Autodesk Inventor part; units mm, degrees
ref_plane "YZ Plane" through (0, 0, 0) normal (1, 0, 0) x (0, 1, 0)
ref_plane "XZ Plane" through (0, 0, 0) normal (0, 1, 0) x (-1, 0, 0)
ref_plane "XY Plane" through (0, 0, 0) normal (0, 0, 1) x (1, 0, 0)
sketch "スケッチ1" plane through (0, 0, 0) normal (0, 0, 1) x (1, 0, 0)
  circle A0 centre (0, 0) radius 48.5
  circle A1 centre (0, 0) radius 46
  dimension "d0" = 97
  dimension "d1" = 92
extrude "押し出し1" add sketch "スケッチ1" along normal blind 20.5 contours A0 | A1
sketch "スケッチ2" plane through (0, 0, 20.5) normal (0, 0, 1) x (1, 0, 0)
  circle A0 centre (0, 0) radius 46
  line L0 (0, 0) -> (0, 59.211017)
  line L1 (0, 0) -> (-21.860946, 52.776992)
  line L2 (0, 0) -> (27.822621, 47.858094)
  point P0 (-17.603438, 42.498458)
  point P1 (-42.498458, 17.603438)
  point P2 (-42.498458, -17.603438)
  point P3 (-17.603438, -42.498458)
  point P4 (17.603438, -42.498458)
  point P5 (42.498458, -17.603438)
  point P6 (42.498458, 17.603438)
  point P7 (17.603438, 42.498458)
  dimension "d4" = 92
  dimension "d5" = 22.5
  dimension "d8" = 360
hole "穴1" at (-17.603438, 42.498458, 20.5) at (-42.498458, 17.603438, 20.5) at (-42.498458, -17.603438, 20.5) at (-17.603438, -42.498458, 20.5) at (17.603438, -42.498458, 20.5) at (42.498458, -17.603438, 20.5) at (42.498458, 17.603438, 20.5) at (17.603438, 42.498458, 20.5) direction (0, 0, -1) diameter 2.459 end through all
sketch "スケッチ3" plane through (0, 0, 20.5) normal (0, 0, 1) x (1, 0, 0)
  circle A0 centre (0, 0) radius 43.5
  dimension "d17" = 87
extrude "押し出し2" cut sketch "スケッチ3" against normal blind 20
sketch "スケッチ4" plane through (0, 0, 0) normal (0, 0, -1) x (-1, 0, 0)
  line L0 (0, 0) -> (0, -80.557014)
  circle A0 centre (0, 0) radius 48.5
  line L1 (-29.457728, -38.529109) -> (145.313488, -172.151794)
  line L2 (29.457728, 38.529109) -> (204.228945, -95.093576)
  line L3 (145.313488, -172.151794) -> (204.228945, -95.093576)
  point P0 (29.457728, 38.529109)
  dimension "d21" = 48.5
  dimension "d23" = 97
  dimension "d24" = 220
  dimension "d25" = 220
  dimension "d56" = 52.6
extrude "押し出し3" add sketch "スケッチ4" against normal blind 5 contours A0 L2 L3 L1 L0 | L0 L1 A0
sketch "スケッチ5" plane through (0, 0, 5) normal (0, 0, 1) x (1, 0, 0)
  line L0 (-29.457728, 38.529109) -> (29.457728, -38.529109)
  line L1 (-204.228945, -95.093576) -> (-145.313488, -172.151794)
  line L2 (29.457728, -38.529109) -> (-145.313488, -172.151794)
  line L3 (-145.313488, -172.151794) -> (-204.228945, -95.093576)
  line L4 (-204.228945, -95.093576) -> (-29.457728, 38.529109)
  line L5 (-26.420849, 34.557036) -> (-201.192066, -99.065649)
  line L6 (26.420849, -34.557036) -> (-148.350367, -168.179721)
  line L7 (-200.256872, -92.056696) -> (-141.341415, -169.114915)
  circle A0 centre (0, 0) radius 48.5
  circle A1 centre (0, 0) radius 43.5
  point P0 (-116.843336, -28.282233)
  point P1 (-60.964759, -101.368378)
  point P2 (-57.92788, -105.340451)
  point P3 (-174.771217, -133.622685)
  point P4 (-170.799143, -130.585806)
  point P5 (-174.771217, -133.622685)
  point P6 (-43.459144, 21.530276)
  point P7 (9.382554, -47.583796)
  point P8 (-144.378294, -165.142842)
  point P9 (-197.219992, -96.02877)
  dimension "d29" = 5
  dimension "d30" = 5
  dimension "d32" = 5
  dimension "d33" = 5
extrude "押し出し4" add sketch "スケッチ5" along normal blind 15.5 contours A0 L5 L7 L4 | L7 L5 L1 L4 | L7 L6 L1 L5 | L2 L7 L6 A0 | L7 L2 L1 L6
sketch "スケッチ6" plane through (0, 0, 20.5) normal (0, 0, 1) x (1, 0, 0)
  line L0 (-204.228945, -95.093576) -> (-145.313488, -172.151794)
  arc A0 (29.457728, -38.529109) -> (-29.457728, 38.529109) centre (0, 0) ccw
  line L1 (-29.457728, 38.529109) -> (-204.228945, -95.093576)
  line L2 (-145.313488, -172.151794) -> (29.457728, -38.529109)
  point P0 (-15.753516, -69.948744)
  point P1 (-71.632093, 3.137401)
  point P2 (-59.44632, -103.354415)
  point P3 (-115.324897, -30.26827)
  point P4 (-103.139124, -136.760086)
  point P5 (-159.017701, -63.673941)
  point P6 (-174.771217, -133.622685)
  point P7 (38.529109, 29.457728)
  point P8 (9.382554, -47.583796)
  dimension "d36" = 268.5
  dimension "d37" = 55
  dimension "d38" = 55
  dimension "d39" = 55
  dimension "d40" = 2.5
  dimension "d41" = 2.5
  dimension "d42" = 2.5
  dimension "d43" = 55
  dimension "d44" = 55
  dimension "d45" = 55
  dimension "d46" = 2.5
  dimension "d47" = 2.5
  dimension "d48" = 2.5
hole "穴2" at (-15.753516, -69.948744, 20.5) at (-71.632093, 3.137401, 20.5) at (-59.44632, -103.354415, 20.5) at (-115.324897, -30.26827, 20.5) at (-103.139124, -136.760086, 20.5) at (-159.017701, -63.673941, 20.5) direction (0, 0, -1) diameter 2.459 end through all
sketch "スケッチ7" plane through (0, 0, 5) normal (0, 0, 1) x (1, 0, 0)
  line L0 (9.382554, -47.583796) -> (-144.378294, -165.142842)
  line L1 (-144.378294, -165.142842) -> (-197.219992, -96.02877)
  point P0 (0, 0)
  point P1 (-135.730252, -127.061201)
  dimension "d57" = 25
  dimension "d58" = 30
hole "穴3" at (-135.730252, -127.061201, 5) direction (0, 0, -1) diameter 5 end through all
sketch "スケッチ8" plane through (0, 0, 5) normal (0, 0, 1) x (1, 0, 0)
  line L0 (-204.228945, -95.093576) -> (-29.457728, 38.529109)
  line L1 (29.457728, -38.529109) -> (-145.313488, -172.151794)
  line L2 (-204.228945, -95.093576) -> (-145.313488, -172.151794)
  line L3 (-145.313488, -172.151794) -> (-204.228945, -95.093576)
  line L4 (29.457728, -38.529109) -> (-145.313488, -172.151794)
  arc A0 (-43.459144, 21.530276) -> (9.382554, -47.583796) centre (0, 0) ccw
  line L5 (-43.459144, 21.530276) -> (-176.491161, -123.140956)
  line L6 (-197.219992, -96.02877) -> (-144.378294, -165.142842)
  line L7 (-47.512963, 9.734903) -> (-173.407433, -127.174304)
  dimension "d66" = 80
  dimension "d67" = 5
extrude "押し出し5" add sketch "スケッチ8" along normal blind 10
sketch "スケッチ9" plane through (0, 0, 20.5) normal (0, 0, 1) x (1, 0, 0)
  circle A0 centre (0, 0) radius 48.5
  line L0 (-29.457728, 38.529109) -> (-204.228945, -95.093576)
  line L1 (-29.457728, 38.529109) -> (-204.228945, -95.093576)
  line L2 (-204.228945, -95.093576) -> (-144.905471, -172.685458)
  line L3 (-43.459144, 21.530276) -> (-179.92775, -126.878218)
  line L4 (-43.459144, 21.530276) -> (-176.491161, -123.140956)
  dimension "d70" = 97
  dimension "d71" = 80
  dimension "d72" = 0
sketch "スケッチ9 outline for 押し出し6" plane through (0, 0, 20.5) normal (0, 0, 1) x (1, 0, 0)
  line L0 (-179.92775, -126.878218) -> (-43.459144, 21.530276)
  line L1 (-204.228945, -95.093576) -> (-179.92775, -126.878218)
  line L2 (-29.457728, 38.529109) -> (-204.228945, -95.093576)
  arc A0 (-43.459144, 21.530276) -> (-29.457728, 38.529109) centre (0, 0) cw
extrude "押し出し6" cut sketch "スケッチ9 outline for 押し出し6" against normal through all
sketch "スケッチ10" plane through (0, 0, 20.5) normal (0, 0, 1) x (1, 0, 0)
  line L0 (-47.512963, 9.734903) -> (-173.407433, -127.174304)
  line L1 (-65.245855, -9.549472) -> (-68.329583, -5.516124)
  line L2 (-176.491161, -123.140956) -> (-179.92775, -126.878218)
  line L3 (-144.378294, -165.142842) -> (-173.407433, -127.174304)
  line L4 (-173.407433, -127.174304) -> (-176.527747, -123.093103)
  line L5 (-158.56619, -111.034574) -> (-161.649918, -107.001226)
  line L6 (-68.329583, -5.516124) -> (-161.649918, -107.001226)
  line L7 (-158.56619, -111.034574) -> (-65.245855, -9.549472)
  circle A0 centre (0, 0) radius 48.5
  line L8 (-43.459144, 21.530276) -> (-68.329583, -5.516124)
  line L9 (-47.512963, 9.734903) -> (-65.245855, -9.549472)
  line L10 (-158.56619, -111.034574) -> (-173.407433, -127.174304)
  line L11 (-144.378294, -165.142842) -> (-173.407433, -127.174304)
  line L12 (-179.92775, -126.878218) -> (-145.069701, -172.470655)
  line L13 (-144.378294, -165.142842) -> (9.382554, -47.583796)
  line L14 (-145.069701, -172.470655) -> (-81.516531, -123.880587)
  line L15 (-161.649918, -107.001226) -> (-179.92775, -126.878218)
  line L16 (-81.516531, -123.880587) -> (-84.797198, -119.589654)
  line L17 (9.382554, -47.583796) -> (9.382554, -42.583206)
  line L18 (-35.700709, 32.828485) -> (-32.020223, 29.444105)
  circle A1 centre (0, 0) radius 43.5
  circle A2 centre (0, 0) radius 43.5
  dimension "d75" = 97
  dimension "d78" = 80
  dimension "d79" = 87
  dimension "d80" = 5
extrude "押し出し7" cut sketch "スケッチ10" against normal through all contours L0 L1 L8 A0 | L0 L5 L6 L1 | L0 L4 L15 L5 | L16 L14 L12 L2 L4 L3 L13
sketch "スケッチ11" plane through (0, 0, 20.5) normal (0, 0, 1) x (1, 0, 0)
  circle A0 centre (0, 0) radius 43.5
  circle A1 centre (0, 0) radius 48.5
  line L0 (-22.603438, 42.910775) -> (-22.603438, 37.16631)
  circle A2 centre (-17.603438, 42.498458) radius 1.2295
  arc A3 (-47.512963, 9.734903) -> (9.382554, -47.583796) centre (0, 0) ccw
  line L1 (9.382554, -47.583796) -> (9.382554, -42.476084)
  point P0 (-22.603438, 40.038542)
  dimension "d81" = 87
  dimension "d82" = 97
  dimension "d83" = 5
extrude "押し出し8" cut sketch "スケッチ11" against normal blind 15.5 contours A0 L1 A1 L0 picked at (-35.223195, -30.551112)
equation "\"d25\" = d24"
properties part number "legparts_05"
Part model, mm, in its own coordinate system. A direction names the side the tool comes from. Round coordinates to 2 decimals unless told otherwise and drop trailing zeros. Order: outer loops, then holes, each group sorted by start corner. A loop starts at its lowest first (then second) coordinate and runs counter-clockwise, first axis right, second up. Notation, with made-up numbers: M 12,51 L 36,51 A24 ccw 36,61 Z; hole C 75,51.25 d5. An arc over 180 degrees is marked long. Put each result on its own line as item: value. Start each with the question number.
1. Slice it at A-A on z = 9. List the corners of the cut face in (x, y).
2. Drill centre lines: probe 1 along Y at (x, z) = (17, 12.5); probe 2 along Z at (x, y) = (-104, -94); probe 3 along Z at (x, y) = (10.5, 35.5). Where is each one in solid material? Low to high. Write a range as [from, to].
3. Slice it at C-C on x = 0. List the corners of the cut face in (y, z).
4. Slice it at D-D on y = -28.5. List the corners of the cut face in (x, z).
5. Drop flat-ended pins along their axis: pin 1 (4.5 mm diameter, centred on y = 40.5, z = 14, fed in from -X); pin 2 (12 mm diameter, centred on y = -56, z = 10, fed in from -X); pin 3 (1 mm diameter, centred on y = -76.5, z = 7.5, fed in from -X). Give the stop position or say it passes through.
6. Two-plate mould, pull along Y, no slides. Class faces 1 (the face through (-158.69, -146.424, 2.535)), 2 (the face through (-137.4, -125.2, 2.5)), 3 (the face through (-39, -57, 0)): +Y half, -Y half, draft (parallel to the pull), parting line (faces both ways), or undercut.
7. Tool access for faces 4 (the face through (-22.603, 40, 13)), 5 (the face through (-37.048, -83.083, 12.642)), 6 (the face through (41.49, 13.07, 8.42)), 7 (the face through (-25.37, -80.45, 10.11)), 8 (the face through (11, -44, 20.5)): list every direction of +Z, -Z, +X, -X, +Y, -Y with a clear straight run to the whole face (end or side of a thin tool).
8. Slice it at B-B on y = -86. List the corners of the cut face in (x, z), then the cut area to 3 significant figures.
Findings:
1. outline: M -84.8,-119.59 L -81.76,-123.56 L 29.46,-38.53 A48.5 ccw -22.6,42.91 L -22.6,37.17 A43.5 cw long 9.38,-42.48 L 9.38,-47.58 Z; hole C -59.45,-103.35 d2.46; hole C -17.6,42.5 d2.46; hole C -15.75,-69.95 d2.46; hole C 17.6,-42.5 d2.46; hole C 17.6,42.5 d2.46; hole C 42.5,-17.6 d2.46; hole C 42.5,17.6 d2.46
2. probe 1: [-48.05, -43.57], [-41.43, -40.04], [40.04, 41.43], [43.57, 45.42]
2. probe 2: [0, 5]
2. probe 3: [0, 0.5]
3. outline: M -61.05,0 L 48.5,0 L 48.5,20.5 L 43.5,20.5 L 43.5,0.5 L -43.5,0.5 L -43.5,5 L -54.76,5 L -54.76,20.5 L -61.05,20.5 Z
4. outline: M -82.67,0 L 39.24,0 L 39.24,20.5 L 32.86,20.5 L 32.86,0.5 L -32.86,0.5 L -32.86,5 L -82.67,5 Z
5. pin 1: x = -22.6
5. pin 2: x = -111.01
5. pin 3: x = -29.09
6. face 1: -Y half
6. face 2: undercut
6. face 3: draft
7. face 4: +Z, -X, +Y
7. face 5: +Z, -X
7. face 6: +Z
7. face 7: +Z, -Z, +X, -Y
7. face 8: +Z, +X, -X, +Y, -Y
8. outline: M -135.55,0 L -32.63,0 L -32.63,20.5 L -40.86,20.5 L -40.86,5 L -135.55,5 Z
8. area: 642 mm2
